```python
from build123d import *

# Parameters (mm, degrees)
BOSS_EXTRU_1_DEPTH      = 3
CONG_1_R                = 3
ESQUISSE2_R             = 3
PER_AGE_PROFIL_DEPTH    = 4
ESQUISSE3_R             = 3
ENL_V_MAT_EXTRU_1_DEPTH = 4
ENL_V_MAT_EXTRU_3_REACH = 5
ESQUISSE5_R             = 1.7
ENL_V_MAT_EXTRU_4_REACH = 5
CONG_2_R                = 2
ENL_V_MAT_EXTRU_2_REACH = 5


with BuildPart() as part:
    # Esquisse1 → Boss.-Extru.1 (new body)
    with BuildSketch(Plane(origin=(0, 0, 0), x_dir=(1, 0, 0), z_dir=(0, 1, 0))):
        Polygon((-130, 125), (130, 125), (155, 100), (155, -100), (130, -125), (-130, -125), (-155, -100), (-155, 100), align=None)
    extrude(amount=BOSS_EXTRU_1_DEPTH)

    # Congé1
    cong_1_edges = [part.edges().sort_by_distance(p)[0] for p in [
        (155, 1.5, -100),
        (155, 1.5, 100),
        (130, 1.5, 125),
        (-130, 1.5, 125),
        (-155, 1.5, 100),
        (-155, 1.5, -100),
        (-130, 1.5, -125),
        (130, 1.5, -125),
    ]]
    fillet(cong_1_edges, radius=CONG_1_R)

    # Esquisse2 → Perçage Profilé (cut, through all)
    with BuildSketch(Plane(origin=(0, 3, 0), x_dir=(1, 0, 0), z_dir=(0, 1, 0))):
        with Locations((-132, 65)):
            Circle(ESQUISSE2_R)
        with Locations((-132, -65)):
            Circle(ESQUISSE2_R)
        with Locations((132, -65)):
            Circle(ESQUISSE2_R)
        with Locations((132, 65)):
            Circle(ESQUISSE2_R)
    extrude(amount=-PER_AGE_PROFIL_DEPTH, mode=Mode.SUBTRACT)

    # Esquisse3 → Enlèv. mat.-Extru.1 (cut, through all)
    with BuildSketch(Plane(origin=(0, 3, 0), x_dir=(1, 0, 0), z_dir=(0, 1, 0))):
        with Locations((-36.5, -52)):
            Circle(ESQUISSE3_R)
        with Locations((36.5, -52)):
            Circle(ESQUISSE3_R)
    extrude(amount=-ENL_V_MAT_EXTRU_1_DEPTH, mode=Mode.SUBTRACT)

    # Esquisse5 → Enlèv. mat.-Extru.3 (cut, up to next)
    with BuildSketch(Plane(origin=(0, 3, 0), x_dir=(1, 0, 0), z_dir=(0, 1, 0)), mode=Mode.PRIVATE) as enl_v_mat_extru_3_sk1:
        with Locations((0, -35.89)):
            Circle(ESQUISSE5_R)
    enl_v_mat_extru_3_tool1 = extrude(enl_v_mat_extru_3_sk1.sketch, amount=-ENL_V_MAT_EXTRU_3_REACH, mode=Mode.PRIVATE) & part.part
    add(enl_v_mat_extru_3_tool1.solids().sort_by_distance((0, 3, 35.89))[0], mode=Mode.SUBTRACT)
    # Esquisse5 → Enlèv. mat.-Extru.3 (cut, up to next)
    with BuildSketch(Plane(origin=(0, 3, 0), x_dir=(1, 0, 0), z_dir=(0, 1, 0)), mode=Mode.PRIVATE) as enl_v_mat_extru_3_sk2:
        with Locations((39, 3.11)):
            Circle(ESQUISSE5_R)
    enl_v_mat_extru_3_tool2 = extrude(enl_v_mat_extru_3_sk2.sketch, amount=-ENL_V_MAT_EXTRU_3_REACH, mode=Mode.PRIVATE) & part.part
    add(enl_v_mat_extru_3_tool2.solids().sort_by_distance((39, 3, -3.11))[0], mode=Mode.SUBTRACT)

    # Esquisse6 → Enlèv. mat.-Extru.4 (cut, up to next)
    with BuildSketch(Plane(origin=(0, 3, 0), x_dir=(1, 0, 0), z_dir=(0, 1, 0)), mode=Mode.PRIVATE) as enl_v_mat_extru_4_sk1:
        with BuildLine():
            Line((-20, 33), (20, 33))
            Line((20, 33), (20, 17))
            ThreePointArc((20, 17), (0, 14.523581408), (-20, 17))
            Line((-20, 17), (-20, 33))
        make_face()
    enl_v_mat_extru_4_tool1 = extrude(enl_v_mat_extru_4_sk1.sketch, amount=-ENL_V_MAT_EXTRU_4_REACH, mode=Mode.PRIVATE) & part.part
    add(enl_v_mat_extru_4_tool1.solids().sort_by_distance((0, 3, -24.156632))[0], mode=Mode.SUBTRACT)

    # Congé2
    cong_2_edges = [part.edges().sort_by_distance(p)[0] for p in [
        (-20, 1.5, -17),
        (-20, 1.5, -33),
        (20, 1.5, -33),
        (20, 1.5, -17),
    ]]
    fillet(cong_2_edges, radius=CONG_2_R)

    # Esquisse4 → Enlèv. mat.-Extru.2 (cut, up to next)
    with BuildSketch(Plane(origin=(0, 3, 0), x_dir=(1, 0, 0), z_dir=(0, 1, 0)), mode=Mode.PRIVATE) as enl_v_mat_extru_2_sk1:
        Polygon((122, 55), (-122, 55), (-122, 75), (-128.757359313, 120), (-128.757359313, 125), (128.757359313, 125), (128.757359313, 120), (122, 75), align=None)
    enl_v_mat_extru_2_tool1 = extrude(enl_v_mat_extru_2_sk1.sketch, amount=-ENL_V_MAT_EXTRU_2_REACH, mode=Mode.PRIVATE) & part.part
    add(enl_v_mat_extru_2_tool1.solids().sort_by_distance((0, 3, -90.387205))[0], mode=Mode.SUBTRACT)


solid = part.part
```
Read the model definition and answer for the solid it produces. Units are mm, in the model's axes. A direction names the side the tool comes from. Give positions to 0.01 mm unless a question says otherwise; leave off trailing zeros. Order: outer loops, then holes, each group sorted by start corner. A loop starts at its lowest first (then second) coordinate and runs counter-clockwise, first axis right, second up.
(1) For faces 4 (the flat face through (-125.33, 1.52, -97.18)), 5 (the cylindrical face through (134.77, 1.52, -63.85)), determine the directions among +Z, -Z, +X, -X, +Y, -Y from which every point of the face is accessible in a straight line to the end or side of a thin tool.
(2) Find section D-D (x = -43). Give the vertices of the cut face in (y, z).
(3) Find section A-A (z = -90.5). Give the vertices of the cut face in (x, y).
(4) For a pull along X with two mould halves and no side action, classify faces 1 (the flat face through (-142, 1, 113)), 2 (the cylindrical face through (-38.71, 1.52, 49.97)), 3 (the flat face through (142, 1, -113)) as released by +X, released by -X, zero draft, split by the parting line, or undercut.
(5) Straight lines are drawn through the part: L1, parallel to Z at x = 0, y = 1.85; L2, parallel to X at y = 0.8, z = -3.11; L3, parallel to X at y = 1.4, z = 35.89. For each, find the intervals that lie inside material, in ascending order.
(6) Given pin 1 (1.5 mm diameter, centred on y = 1, z = -122, fed in from +X); pin 2 (1.5 mm diameter, centred on y = 1, z = -121.5, fed in from -X), each flat-ended and moving along its own axis, determine where each tip first touches the part or whether it passes through.
(7) Find section B-B (x = -6.5). Give the vertices of the cut face in (y, z), plus the area to 3 significant figures.
(8) Find section C-C (y = 1.15). Give the number of separate pieces and of enclosed holes in the cut face, plus the area to 3 significant figures.
Result sheet:
1. face 4: -Z, +Y, -Y
1. face 5: +Y, -Y
2. outline: (0, -55) - (3, -55) - (3, 125) - (0, 125) - close
3. outline: (-155, 0) - (-124.33, 0) - (-124.33, 3) - (-155, 3) - close; (124.33, 0) - (155, 0) - (155, 3) - (124.33, 3) - close
4. face 1: released by -X
4. face 2: undercut
4. face 3: released by +X
5. L1: z = -55 to -33, -14.52 to 34.19, 37.59 to 125
5. L2: x = -155 to 37.3, 40.7 to 155
5. L3: x = -155 to -1.7, 1.7 to 155
6. pin 1: stops at x = 133.75
6. pin 2: stops at x = -134.25
7. outline: (0, -55) - (3, -55) - (3, -33) - (0, -33) - close; (0, -14.78) - (3, -14.78) - (3, 125) - (0, 125) - close
7. area: 485 mm2
8. separate pieces: 1
8. enclosed holes: 9
8. area: 57,900 mm2
